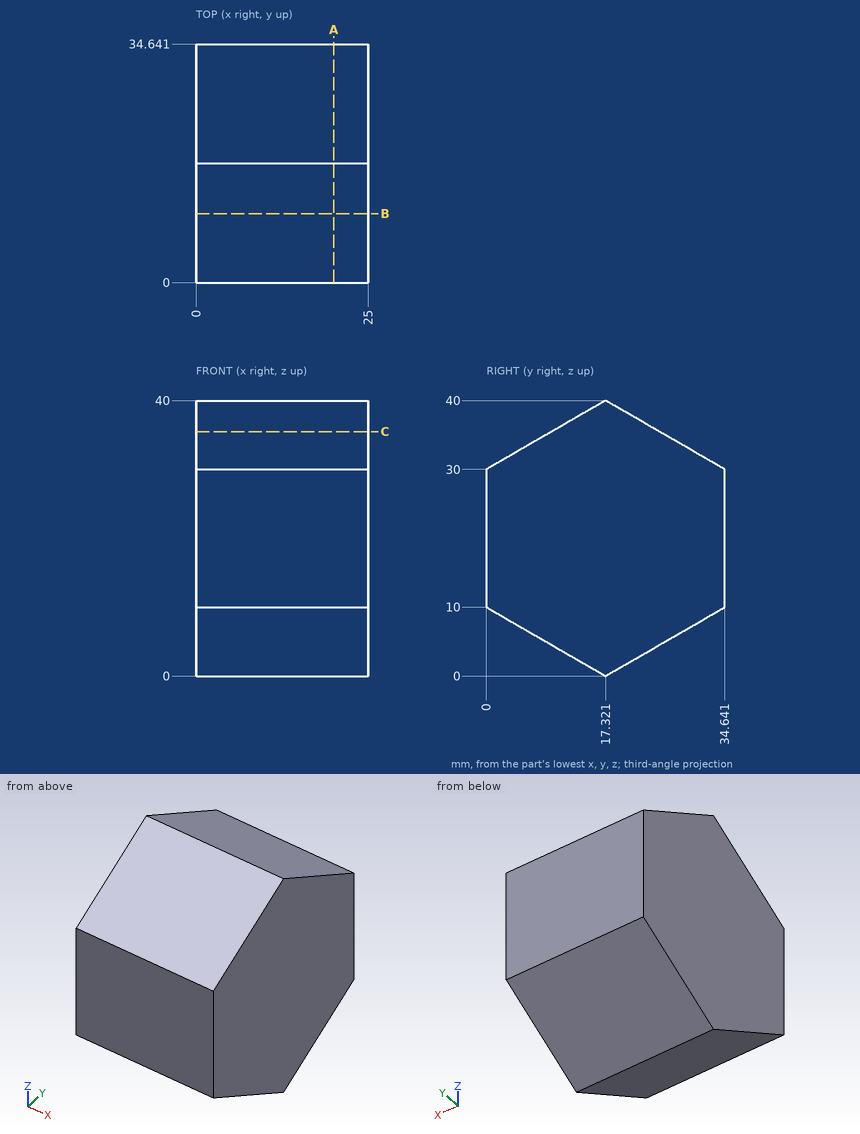
Design review of the part shown in the three views and the two pictorial views. Dimensions are in mm from the part's minimum x, y and z. Give positions to 0.01 mm unless a question says otherwise; leave off trailing zeros. Order: outer loops, then holes, each group sorted by start corner. A loop starts at its lowest first (then second) coordinate and runs counter-clockwise, first axis right, second up. Notation, with made-up numbers: M -39,18 L -15,18 A11 cw -15,23 Z; hole C 84.25,-37 d2. An arc over 180 degrees is marked long. Answer in a Markdown table with one row per item. Add a question column.
(1) For pin 1 (5 mm diameter, centred on x = 15.5, z = 5.5, fed in from +Y) (1 decimal); pin 2 (6 mm diameter, centred on x = 7, y = 10.5, fed in from -Z) (1 decimal); pin 3 (2 mm diameter, centred on x = 5.5, z = 31.5, fed in from -Y) (1 decimal), all flat-tipped, find the tip position at first contact; note any pin that passes through.
(2) Consider section B-B on y = 10. State the section outline as (x, z) points, and give its area (3 significant figures).
(3) Consider section C-C on z = 35.5. State the section outline as (x, y) points (1 decimal).
(4) Wall thickness on probe 1 along Z at (x, y) = (12, 14) (1 decimal); probe 2 along Z at (x, y) = (5.5, 22); probe 3 along Y at (x, z) = (1.25, 32) (1 decimal): over which ranges is each line inside the solid? List them lowest first. Write a range as [from, to].
(5) Consider section A-A on x = 20. State the section outline as (y, z) points.
Evaluation:
| question | item | result |
|---|---|---|
| 1 | pin 1 | stops at y = 31.2 |
| 1 | pin 2 | stops at z = 2.2 |
| 1 | pin 3 | stops at y = 0.9 |
| 2 | outline | M 0,4.23 L 25,4.23 L 25,35.77 L 0,35.77 Z |
| 2 | area | 789 mm^2 |
| 3 | outline | M 0,9.5 L 25,9.5 L 25,25.1 L 0,25.1 Z |
| 4 | probe 1 | z = [1.9, 38.1] |
| 4 | probe 2 | z = [2.7, 37.3] |
| 4 | probe 3 | y = [3.5, 31.2] |
| 5 | outline | M 0,10 L 17.32,0 L 34.64,10 L 34.64,30 L 17.32,40 L 0,30 Z |
